Geometry: final body of the model. Coordinates: model frame, mm. Coordinates: 2 decimals unless noted, no trailing zeros. Order: outer loops, then holes, each group sorted by start corner. A loop starts at its lowest first (then second) coordinate and runs counter-clockwise, first axis right, second up. Notation, with made-up numbers: M 57,34.5 L 63,34.5 A33 cw 63,67.5 Z; hole C 63,-18 d7. An arc over 180 degrees is marked long. Use CSV: the item, a comma, the result in double quotes. Start each with the question number.
1. Section query C-C on z = 74. Return the cut outline in (x, y) (1 decimal), and give its area (3 significant figures).
2. First-contact query: P1, Ø1, axis at y = 2, z = 62, coming from the +X side; P2, Ø4.5, axis at x = 0, y = 0, coming from the -Z side. Flat tips, straight axial feed; report the tip coordinate or a pass-through.
3. Material intervals for line 1 (Y direction, x = 0, z = 36.5); line 2 (Y direction, x = -0.25, z = 24); line 3 (X direction, y = 1.5, z = 56.5), sorted ascending.
4. Section query A-A on y = 0. Return the cut outline in (x, z).
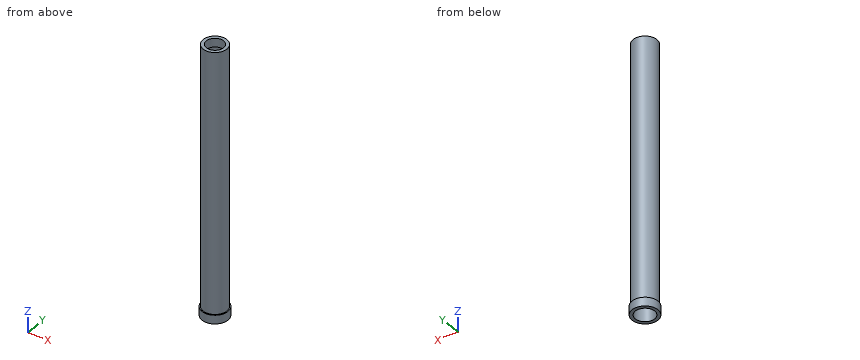
from build123d import *

# Parameters (mm, degrees)
SKETCH1_R           = 3.4925
SKETCH1_R_2         = 2.8575
BOSS_EXTRUDE1_DEPTH = 76.2
SKETCH2_R           = 3.4925
SKETCH2_R_2         = 2.54
BOSS_EXTRUDE2_DEPTH = 2.54
SKETCH3_R           = 3.81
SKETCH3_R_2         = 3.4925
BOSS_EXTRUDE3_DEPTH = 2.54


with BuildPart() as part:
    # Sketch1 → Boss-Extrude1 (new body)
    with BuildSketch(Plane.XY):
        with Locations(Location((0, 0, 0), (0, 0, 180))):
            Circle(SKETCH1_R)
        with Locations(Location((0, 0, 0), (0, 0, 180))):
            Circle(SKETCH1_R_2, mode=Mode.SUBTRACT)
    extrude(amount=BOSS_EXTRUDE1_DEPTH)

    # Sketch2 → Boss-Extrude2 (add)
    with BuildSketch(Plane.XY.offset(76.2)):
        with Locations(Location((0, 0, 0), (0, 0, 180))):
            Circle(SKETCH2_R)
        Circle(SKETCH2_R_2, mode=Mode.SUBTRACT)
    extrude(amount=BOSS_EXTRUDE2_DEPTH)

    # Sketch3 → Boss-Extrude3 (add)
    with BuildSketch(Plane(origin=(0, 0, 0), x_dir=(-1, 0, 0), z_dir=(0, 0, -1))):
        Circle(SKETCH3_R)
        Circle(SKETCH3_R_2, mode=Mode.SUBTRACT)
    extrude(amount=-BOSS_EXTRUDE3_DEPTH)


solid = part.part
Results list:
1,outline,"C 0,0 d7; hole C 0,0 d5.7"
1,area,"12.7 mm²"
2,P1,"stops at x = 3.15"
2,P2,"passes through"
3,line 1,"y = -3.49 to -2.86, 2.86 to 3.49"
3,line 2,"y = -3.48 to -2.85, 2.85 to 3.48"
3,line 3,"x = -3.15 to -2.43, 2.43 to 3.15"
4,outline,"M -3.81,0 L -2.86,0 L -2.86,76.2 L -2.54,76.2 L -2.54,78.74 L -3.49,78.74 L -3.49,2.54 L -3.81,2.54 Z; M 2.54,76.2 L 2.86,76.2 L 2.86,0 L 3.81,0 L 3.81,2.54 L 3.49,2.54 L 3.49,78.74 L 2.54,78.74 Z"
